from build123d import *

# Parameters (mm, degrees)
SKETCH_2_W          = 23.064561435
SKETCH_2_H          = 26
SKETCH_2_R          = 1.1
EXTRUDE_1_DEPTH     = 14.5
SKETCH_3_R          = 33
CUT_EXTRUDE_1_DEPTH = 11.6
SKETCH_4_R          = 3.5
CUT_EXTRUDE_2_DEPTH = 54.268776032
SKETCH_5_W          = 15.2
SKETCH_5_H          = 29
CUT_EXTRUDE_3_DEPTH = 4
FILLET_1_R          = 3
SKETCH_6_R          = 1.1
CUT_EXTRUDE_4_DEPTH = 28.252660471
CHAMFER_1_SIZE      = 1
SKETCH_7_R          = 1.8
CUT_EXTRUDE_5_DEPTH = 1
CUT_EXTRUDE_6_DEPTH = 35.75


with BuildPart() as part:
    # Эскиз2 → Бобышка-Вытянуть1 (new, symmetric)
    with BuildSketch(Plane(origin=(0, 0, 0), x_dir=(1, 0, 0), z_dir=(0, 1, 0))):
        with Locations((31.217719282, 0)):
            Rectangle(SKETCH_2_W, SKETCH_2_H)
        with Locations(Location((23.685438565, 8, 0), (0, 0, 90))):
            Circle(SKETCH_2_R, mode=Mode.SUBTRACT)
        with Locations(Location((23.685438565, -8, 0), (0, 0, 90))):
            Circle(SKETCH_2_R, mode=Mode.SUBTRACT)
    extrude(amount=EXTRUDE_1_DEPTH, both=True)

    # Эскиз3 → Вырез-Вытянуть1 (cut, symmetric)
    with BuildSketch(Plane(origin=(0, 0, 0), x_dir=(1, 0, 0), z_dir=(0, 1, 0))):
        Circle(SKETCH_3_R)
    extrude(amount=CUT_EXTRUDE_1_DEPTH, both=True, mode=Mode.SUBTRACT)

    # Эскиз4 → Вырез-Вытянуть2 (cut, through all)
    with BuildSketch(Plane(origin=(0, 14.5, 0), x_dir=(1, 0, 0), z_dir=(0, 1, 0))):
        with Locations((25, 0)):
            Circle(SKETCH_4_R)
        with BuildLine():
            ThreePointArc((25, -3.5), (21.5, 0), (25, 3.5))
            Line((25, 3.5), (19.685438565, 3.5))
            Line((19.685438565, 3.5), (19.685438565, -3.5))
            Line((19.685438565, -3.5), (25, -3.5))
        make_face()
    extrude(amount=-CUT_EXTRUDE_2_DEPTH, mode=Mode.SUBTRACT)

    # Эскиз5 → Вырез-Вытянуть3 (cut)
    with BuildSketch(Plane(origin=(42.75, 0, 0), x_dir=(0, 0, -1), z_dir=(1, 0, 0))):
        Rectangle(SKETCH_5_W, SKETCH_5_H)
    extrude(amount=-CUT_EXTRUDE_3_DEPTH, mode=Mode.SUBTRACT)

    # Скругление1
    fillet_1_edges = [part.edges().sort_by_distance(p)[0] for p in [
        (19.685438565, -13.05, 13),
        (19.685438565, -13.05, -13),
        (19.685438565, 13.05, 3.5),
        (19.685438565, 13.05, -3.5),
        (19.685438565, -13.05, 3.5),
        (19.685438565, -13.05, -3.5),
        (42.75, 0, 13),
        (19.685438565, 13.05, 13),
        (19.685438565, 13.05, -13),
        (42.75, 0, -13),
    ]]
    fillet(fillet_1_edges, radius=FILLET_1_R)

    # Эскиз6 → Вырез-Вытянуть4 (cut, through all)
    with BuildSketch(Plane(origin=(38.75, 0, 0), x_dir=(0, 0, -1), z_dir=(1, 0, 0))):
        with Locations((0, 6)):
            Circle(SKETCH_6_R)
        with Locations((0, -6)):
            Circle(SKETCH_6_R)
    extrude(amount=-CUT_EXTRUDE_4_DEPTH, mode=Mode.SUBTRACT)

    # Фаска1
    chamfer_1_edges = [part.edges().sort_by_distance(p)[0] for p in [
        (20.564118221, 14.5, 12.121320344),
        (20.564118221, 14.5, 4.378679656),
        (20.564118221, 14.5, -4.378679656),
        (20.564118221, 14.5, -12.121320344),
        (41.871320344, 14.5, -12.121320344),
        (28.5, -14.5, 0),
        (23.842719282, -14.5, -3.5),
        (28.5, 14.5, 0),
        (23.842719282, 14.5, -3.5),
        (42.75, -14.5, -8.8),
        (42.75, 14.5, -8.8),
        (31.217719282, 14.5, -13),
        (31.217719282, -14.5, -13),
        (42.75, -14.5, 8.8),
        (31.217719282, -14.5, 13),
        (19.685438565, -14.5, 8.25),
        (23.842719282, -14.5, 3.5),
        (19.685438565, -14.5, -8.25),
        (41.871320344, -14.5, 12.121320344),
        (20.564118221, -14.5, 12.121320344),
        (20.564118221, -14.5, 4.378679656),
        (20.564118221, -14.5, -4.378679656),
        (20.564118221, -14.5, -12.121320344),
        (41.871320344, -14.5, -12.121320344),
        (19.685438565, 14.5, -8.25),
        (23.842719282, 14.5, 3.5),
        (19.685438565, 14.5, 8.25),
        (31.217719282, 14.5, 13),
        (42.75, 14.5, 8.8),
        (41.871320344, 14.5, 12.121320344),
    ]]
    chamfer(chamfer_1_edges, length=CHAMFER_1_SIZE)

    # Эскиз7 → Вырез-Вытянуть5 (cut)
    with BuildSketch(Plane(origin=(0, 14.5, 0), x_dir=(1, 0, 0), z_dir=(0, 1, 0))):
        with Locations(Location((23.685438565, 8, 0), (0, 0, 270))):
            Circle(SKETCH_7_R)
        with Locations(Location((23.685438565, -8, 0), (0, 0, 270))):
            Circle(SKETCH_7_R)
    cut_extrude_5 = extrude(amount=-CUT_EXTRUDE_5_DEPTH, mode=Mode.SUBTRACT)

    # Зеркальное отражение1: Вырез-Вытянуть5 across plane
    add(cut_extrude_5.mirror(Plane.ZX), mode=Mode.SUBTRACT)

    # Эскиз8 → Вырез-Вытянуть6 (cut)
    with BuildSketch(Plane(origin=(0, 0, 0), x_dir=(0, 0, -1), z_dir=(1, 0, 0))):
        Polygon((1.125833025, 4.05), (2.25166605, 6), (1.125833025, 7.95), (-1.125833025, 7.95), (-2.25166605, 6), (-1.125833025, 4.05), align=None)
        Polygon((1.125833025, -7.95), (2.25166605, -6), (1.125833025, -4.05), (-1.125833025, -4.05), (-2.25166605, -6), (-1.125833025, -7.95), align=None)
    extrude(amount=CUT_EXTRUDE_6_DEPTH, mode=Mode.SUBTRACT)


solid = part.part
Input: part model. Units: mm. Frame: model coordinates. A direction names the side the tool comes from. Give positions to 0.01 mm unless a question says otherwise; leave off trailing zeros. Order: outer loops, then holes, each group sorted by start corner. A loop starts at its lowest first (then second) coordinate and runs counter-clockwise, first axis right, second up. Notation, with made-up numbers: (88.5, 84) -> (94.5, 84) arc R8 ccw to (94.5, 98) -> close; hole circle Ø3 at (-7.5, 73.25). An arc over 180 degrees is marked (long way). Use one line per item in the form item = value.
1) Mould query, pull axis Y, two halves, no side actions, for faces 4 (the cylindrical face through (37.27, -5.07, -0.59)), 5 (the flat face through (42.26, 13.99, -8.82)), 6 (the cylindrical face through (20.588, -12.563, -4.355)). Classes: pulls with the +Y half, pulls with the -Y half, needs draft (parallel to the pull), parting line crosses it, or undercut.
Response values:
face_4 = undercut
face_5 = pulls with the +Y half
face_6 = needs draft
2) Section D-D, the plane z = 8. Return loops of the section in (x, y).
Response values:
outline = (19.69, -13.5) -> (20.69, -14.5) -> (21.89, -14.5) -> (21.89, -13.5) -> (22.59, -13.5) -> (22.59, -11.6) -> (19.69, -11.6) -> close; (19.69, 11.6) -> (22.59, 11.6) -> (22.59, 13.5) -> (21.89, 13.5) -> (21.89, 14.5) -> (20.69, 14.5) -> (19.69, 13.5) -> close; (24.79, -13.5) -> (25.49, -13.5) -> (25.49, -14.5) -> (41.75, -14.5) -> (42.75, -13.5) -> (42.75, 13.5) -> (41.75, 14.5) -> (25.49, 14.5) -> (25.49, 13.5) -> (24.79, 13.5) -> (24.79, 11.6) -> (32.02, 11.6) -> (32.02, -11.6) -> (24.79, -11.6) -> close
3) Reachability of faces 1 (the cylindrical face through (20.541, 12.537, 4.402)), 2 (the flat face through (24, 14, 4)), 3 (the conical face through (21.01, -14.104, -4.787)) from +Z, -Z, +X, -X, +Y, -Y: full face, straight path, thin tool, end or side. Return the list, or none.
Response values:
face_1 = -X, +Y, -Y
face_2 = -X, +Y
face_3 = -X, -Y
4) Line query: probe 1 along X at (y, z) = (-12.2, -8); probe 2 along Y at (x, z) = (22, 5); probe 3 along X at (y, z) = (-5.5, 1.25). Output: solid intervals per line, ascending.
Response values:
probe_1 = 19.69 to 22.59, 24.79 to 42.75
probe_2 = -14.5 to -11.6, 11.6 to 14.5
probe_3 = 35.75 to 38.75
5) Section C-C, the plane x = 31. Return loops of the section in (y, z), and give its area (3 significant figures).
Response values:
outline = (-14.5, -12) -> (-13.5, -13) -> (13.5, -13) -> (14.5, -12) -> (14.5, 12) -> (13.5, 13) -> (-13.5, 13) -> (-14.5, 12) -> close; hole (-11.6, -11.31) -> (11.6, -11.31) -> (11.6, 11.31) -> (-11.6, 11.31) -> close
area = 227 mm^2
6) Section A-A, the plane z = 0. Return loops of the section in (x, y).
Response values:
outline = (28.5, -13.5) -> (29.5, -14.5) -> (38.75, -14.5) -> (38.75, -7.1) -> (35.75, -7.1) -> (35.75, -7.95) -> (33, -7.95) -> (33, -11.6) -> (28.5, -11.6) -> close; (28.5, 11.6) -> (33, 11.6) -> (33, 7.95) -> (35.75, 7.95) -> (35.75, 7.1) -> (38.75, 7.1) -> (38.75, 14.5) -> (29.5, 14.5) -> (28.5, 13.5) -> close; (33, -4.05) -> (35.75, -4.05) -> (35.75, -4.9) -> (38.75, -4.9) -> (38.75, 4.9) -> (35.75, 4.9) -> (35.75, 4.05) -> (33, 4.05) -> close
7) First-contact query: pin 1 Ø3 at (x, z) = (23.69, -8) entering from +Y; pin 2 Ø2 at (x, z) = (23.69, 8) entering from -Y; pin 3 Ø5 at (y, z) = (-1.5, -1) entering from -X; pin 4 Ø1.2 at (y, z) = (-5.5, 1) entering from -X. Flat tips, straight axial feed; report the tip coordinate or a pass-through.
Response values:
pin_1 = 13.5
pin_2 = through
pin_3 = 32.81
pin_4 = 35.75
8) Section B-B, the plane y = -3.25. Return loops of the section in (x, z).
Response values:
outline = (30.33, -13) -> (39.75, -13) arc R3 ccw to (42.75, -10) -> (42.75, -7.6) -> (38.75, -7.6) -> (38.75, 7.6) -> (42.75, 7.6) -> (42.75, 10) arc R3 ccw to (39.75, 13) -> (30.33, 13) arc R33 cw to start
